Could you check a few things on this model? Use its own coordinates, in mm. A direction names the side the tool comes from. Give positions to 0.01 mm unless a question says otherwise; leave off trailing zeros. Loops run counter-clockwise (first coordinate to the right, second up) from the corner with the lowest first, then second, coordinate; pieces in that order, holes last. Notation, with made-up numbers: (-23.5, 46.25) - (-12.5, 46.25) arc R26 ccw to (-12.5, 65.25) - close; hole circle Ø1 at (1.5, -20.75). An arc over 180 degrees is marked (long way). One line per item, written item: value. Start each with the question number.
Q1. I'm going to push flat-ended pins straight in: P1, Ø8, axis at x = 3.5, z = -2.5, coming from the -Y side; P2, Ø13, axis at y = 79, z = 10.5, coming from the -X side; P3, Ø13, axis at y = 77.5, z = 5.5, coming from the +X side; P4, Ø9.5, axis at x = 3, y = 80, coming from the -Z side. Where does each tip first touch, or does it pass through?
Q2. I want a section at B-B (z = 8). Please give me the cut outline in (x, y) (3 decimals), then the cut area to 3 significant figures.
Q3. If I drill on line 1 (Y direction, x = -6, z = -1); line 2 (Z direction, x = 3, y = 73); line 3 (Y direction, x = -3.5, z = 4), over which ranges is the centre line in solid material (lowest first)? Write a range as from..to.
Q4. I want a section at A-A (x = 0). Please give me the cut outline in (y, z) (3 decimals).
Q5. I want a section at C-C (z = -14.5). Please give me the cut outline in (x, y), then the cut area to 3 significant figures.
Q6. For faces 1 (the face through (-6, 80, 8)), 2 (the face through (0, 80, 14)), 3 (the face through (6, 80, 8)), 4 (the face through (0, 80, 2)), which set-ups out of +Z, -Z, +X, -X, +Y, -Y let a thin tool reach every point of the face, with its end or its side?
```python
from build123d import *

# Parameters (mm, degrees)
SKETCH1_W           = 20
SKETCH1_H           = 36
BOSS_EXTRUDE1_DEPTH = 70
SKETCH2_W           = 12
SKETCH2_H           = 12
BOSS_EXTRUDE2_DEPTH = 20
SKETCH3_R           = 4.445
BOSS_EXTRUDE3_DEPTH = 48


with BuildPart() as part:
    # Sketch1 → Boss-Extrude1 (new body)
    with BuildSketch(Plane(origin=(0, 0, 0), x_dir=(1, 0, 0), z_dir=(0, 1, 0))):
        Rectangle(SKETCH1_W, SKETCH1_H)
    extrude(amount=BOSS_EXTRUDE1_DEPTH)

    # Sketch2 → Boss-Extrude2 (add)
    with BuildSketch(Plane(origin=(0, 70, 0), x_dir=(1, 0, 0), z_dir=(0, 1, 0))):
        with Locations((0, -8)):
            Rectangle(SKETCH2_W, SKETCH2_H)
    extrude(amount=BOSS_EXTRUDE2_DEPTH)

    # Sketch3 → Boss-Extrude3 (add)
    with BuildSketch(Plane(origin=(0, 90, 0), x_dir=(1, 0, 0), z_dir=(0, 1, 0))):
        with Locations((0, -8)):
            Circle(SKETCH3_R)
    extrude(amount=BOSS_EXTRUDE3_DEPTH)


solid = part.part
```
Worked answers:
1. P1: stops at y = 0
1. P2: stops at x = -6
1. P3: stops at x = 6
1. P4: stops at z = 2
2. outline: (-10, 0) - (10, 0) - (10, 70) - (6, 70) - (6, 90) - (4.445, 90) - (4.445, 138) - (-4.445, 138) - (-4.445, 90) - (-6, 90) - (-6, 70) - (-10, 70) - close
2. area: 2,070 mm²
3. line 1: y = 0..70
3. line 2: z = 2..14
3. line 3: y = 0..90
4. outline: (0, -18) - (70, -18) - (70, 2) - (90, 2) - (90, 3.555) - (138, 3.555) - (138, 12.445) - (90, 12.445) - (90, 14) - (70, 14) - (70, 18) - (0, 18) - close
5. outline: (-10, 0) - (10, 0) - (10, 70) - (-10, 70) - close
5. area: 1,400 mm²
6. face 1: +Z, -Z, -X, +Y
6. face 2: +Z, +X, -X, +Y
6. face 3: +Z, -Z, +X, +Y
6. face 4: -Z, +X, -X, +Y
